Geometry: see drawing. Coordinates: mm, zero at the bounding-box minimum. A direction names the side the tool comes from. Give positions to 0.01 mm unless a question says otherwise; leave off trailing zeros. Loops run counter-clockwise (first coordinate to the right, second up) from the corner with the lowest first, then second, coordinate; pieces in that order, holes last. Notation, with made-up numbers: (-31, 7) -> (13, 7) arc R28 ccw to (13, 46) -> close; hole circle Ø5 at (42.5, 67). An arc over 180 degrees is marked (long way). Return JSON: item names as keys, results as strings. Group by question number.
(1) Cut plane C-C on z = 20. Return loops of the section in (x, y).
(2) Cut plane B-B on y = 15. Return loops of the section in (x, z), then the cut area to 3 significant figures.
(3) Ray query, line 1 (Y direction, x = 12.5, z = 0.6); line 2 (X direction, y = 22.5, z = 1.4); line 3 (Z direction, x = 7.75, y = 16.5). Return the intervals inside material, ascending. Write a range as from..to.
(4) Cut plane D-D on x = 3.5. Return loops of the section in (y, z), then the cut area to 3 significant figures.
(5) Pin query (flat end, axial travel): pin 1 (8 mm diameter, centred on x = 8.5, y = 24.5, fed in from +Z); pin 2 (4 mm diameter, centred on y = 6, z = 19, fed in from -X). Return the tip coordinate at first contact, or that it passes through.
(6) Draft query along Y for the marked faces 3, 4 and 5. Return one class per face: released by +Y, released by -Y, zero draft, split by the parting line, or undercut.
(7) Access query for the marked faces 1 and 2. Directions: +Z, -Z, +X, -X, +Y, -Y. A direction counts if a zero-diameter tool reaches every point of the face in a straight line with its end or side. Return the directions, or none.
(8) Cut plane A-A on z = 11.5. Return loops of the section in (x, y).
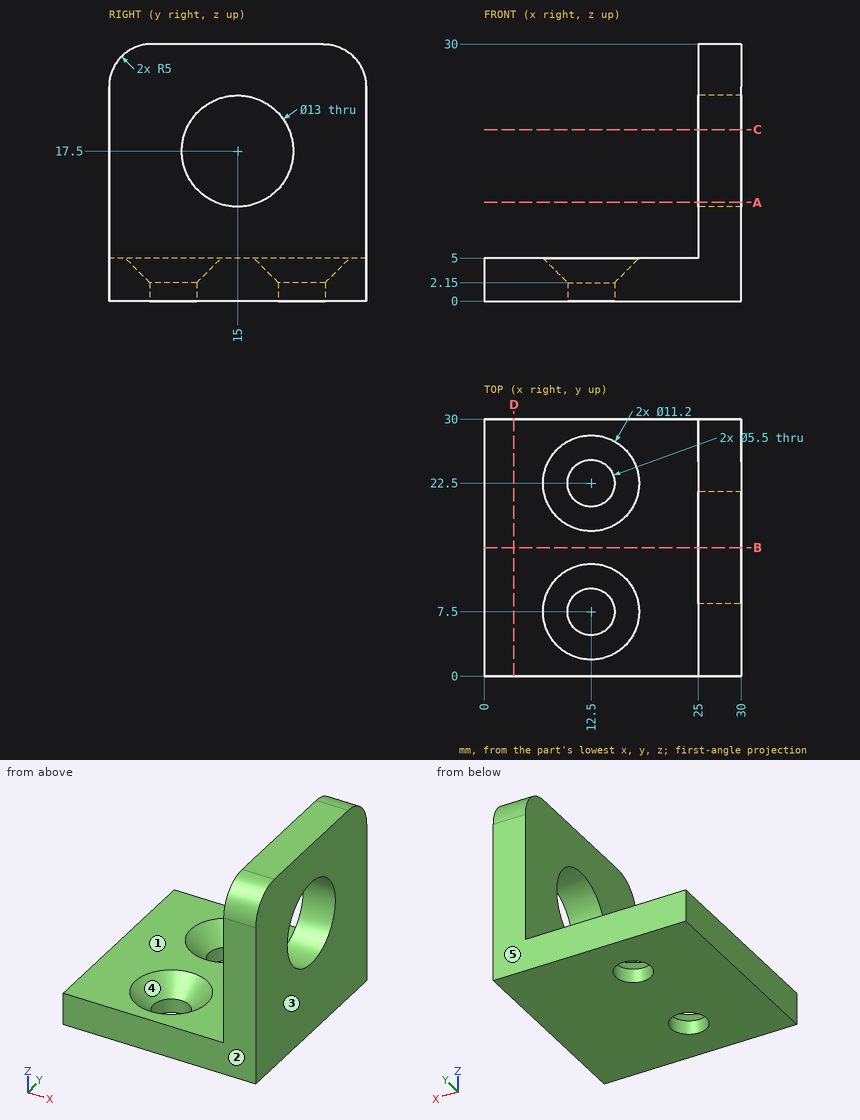
Answers:
{
 "1": {"outline": "(25, 0) -> (30, 0) -> (30, 9) -> (25, 9) -> close; (25, 21) -> (30, 21) -> (30, 30) -> (25, 30) -> close"},
 "2": {"outline": "(0, 0) -> (30, 0) -> (30, 11) -> (25, 11) -> (25, 5) -> (0, 5) -> close; (25, 24) -> (30, 24) -> (30, 30) -> (25, 30) -> close", "area": "210 mm²"},
 "3": {"line 1": "0..4.75, 10.25..19.75, 25.25..30", "line 2": "0..9.75, 15.25..30", "line 3": "0..5"},
 "4": {"outline": "(0, 0) -> (30, 0) -> (30, 5) -> (0, 5) -> close", "area": "150 mm²"},
 "5": {"pin 1": "z = 5", "pin 2": "x = 25"},
 "6": {"face 3": "zero draft", "face 4": "undercut", "face 5": "released by +Y"},
 "7": {"face 1": "+Z, -X, +Y, -Y", "face 2": "+Z, -Z, +X, -X, -Y"},
 "8": {"outline": "(25, 0) -> (30, 0) -> (30, 12.5) -> (25, 12.5) -> close; (25, 17.5) -> (30, 17.5) -> (30, 30) -> (25, 30) -> close"}
}
